```python
from build123d import *

# Parameters (mm, degrees)
PAD011_DEPTH            = 3
FILLET036_R             = 3.35
SKETCH183_R             = 1.15
POCKET052_DEPTH         = 3
POCKET054_DEPTH         = 5
SKETCH187_W             = 31
SKETCH187_H             = 20
POCKET055_DEPTH         = 1.5
BODY023_ROLL_ANGLE      = 180
BODY023_PLACEMENT_ANGLE = -90


with BuildPart() as part:
    # Sketch182 → Pad011 (new body)
    with BuildSketch(Plane(origin=(0, 0, 0), x_dir=(1, 0, 0), z_dir=(0, 0, -1))):
        Polygon((101.467362, -402.500006), (130.400002, -402.500006), (135.400002, -402.500006), (135.400002, -397.500006), (174.999975, -357.90402), (174.999975, -245), (289.999995, -245), (294.999995, -245), (294.999995, -215), (289.999995, -215), (224.999995, -215), (224.999995, -199.999997), (219.999995, -199.999997), (199.999995, -199.999997), (194.999995, -199.999997), (194.999995, -215.000003), (168.459985, -215.000003), (161.999993, -198.359996), (161.999993, -115.000006), (161.999993, -110.000006), (156.999993, -110.000006), (134.576923, -122.534363), (131.999997, -126.895911), (131.999997, -200.027011), (144.989344, -239.967928), (144.989344, -343.839368), (96.467362, -392.500006), (96.467362, -397.500006), (96.467362, -402.500006), align=None)
    extrude(amount=PAD011_DEPTH)

    # Fillet036
    fillet036_edges = [part.edges().sort_by_distance(p)[0] for p in [
        (194.999995, 215.000003, -1.5),
        (168.459985, 215.000003, -1.5),
        (161.999993, 198.359996, -1.5),
        (161.999993, 110.000006, -1.5),
        (156.999993, 110.000006, -1.5),
        (134.576923, 122.534363, -1.5),
        (131.999997, 126.895911, -1.5),
        (131.999997, 200.027011, -1.5),
        (144.989344, 239.967928, -1.5),
        (144.989344, 343.839368, -1.5),
        (96.467362, 392.500006, -1.5),
        (135.400002, 397.500006, -1.5),
        (174.999975, 357.90402, -1.5),
        (174.999975, 245, -1.5),
        (294.999995, 245, -1.5),
        (294.999995, 215, -1.5),
        (224.999995, 215, -1.5),
    ]]
    fillet(fillet036_edges, radius=FILLET036_R)

    # Sketch183 (on Face5 of Fillet036) → Pocket052 (cut)
    with BuildSketch(Plane(origin=(0, 0, -3), x_dir=(1, 0, 0), z_dir=(0, 0, -1))):
        with Locations((105, -389)):
            Circle(SKETCH183_R)
        with Locations((145, -349)):
            Circle(SKETCH183_R)
        with Locations((147.500002, -309.000005)):
            Circle(SKETCH183_R)
        with Locations((147.500002, -259.000004)):
            Circle(SKETCH183_R)
        with Locations((172.500003, -259.000004)):
            Circle(SKETCH183_R)
        with Locations((172.500003, -309.000005)):
            Circle(SKETCH183_R)
        with Locations((172.500003, -349.000005)):
            Circle(SKETCH183_R)
        with Locations((147.665007, -382.765018)):
            Circle(SKETCH183_R)
        with Locations((178.000003, -242.500004)):
            Circle(SKETCH183_R)
        with Locations((218.000003, -242.500004)):
            Circle(SKETCH183_R)
        with Locations((258.000004, -242.500004)):
            Circle(SKETCH183_R)
        with Locations((258.000004, -217.500003)):
            Circle(SKETCH183_R)
        with Locations((292, -242.500004)):
            Circle(SKETCH183_R)
        with Locations((292.000004, -217.500003)):
            Circle(SKETCH183_R)
        with Locations((292.500004, -230.000003)):
            Circle(SKETCH183_R)
        with Locations((223.000003, -217.000003)):
            Circle(SKETCH183_R)
        with Locations((197, -217)):
            Circle(SKETCH183_R)
        with Locations((166.109996, -217.109995)):
            Circle(SKETCH183_R)
        with Locations((147.500002, -239)):
            Circle(SKETCH183_R)
        with Locations((141, -220)):
            Circle(SKETCH183_R)
        with Locations((134.427551, -201)):
            Circle(SKETCH183_R)
        with Locations((160.149996, -200.999996)):
            Circle(SKETCH183_R)
        with Locations((134.427551, -161)):
            Circle(SKETCH183_R)
        with Locations((159.500002, -161.000002)):
            Circle(SKETCH183_R)
        with Locations((137, -124)):
            Circle(SKETCH183_R)
        with Locations((146.849997, -118.149997)):
            Circle(SKETCH183_R)
        with Locations((159, -113)):
            Circle(SKETCH183_R)
    extrude(amount=-POCKET052_DEPTH, mode=Mode.SUBTRACT)

    # Sketch186 (on Face5 of Pocket052) → Pocket054 (cut)
    with BuildSketch(Plane(origin=(0, 0, -3), x_dir=(1, 0, 0), z_dir=(0, 0, -1))):
        Polygon((175, -249), (130, -249), (130, -100), (170, -100), (170, -190), (300, -190), (300, -249), align=None)
    extrude(amount=-POCKET054_DEPTH, mode=Mode.SUBTRACT)

    # Sketch187 (on Face25 of Pocket054) → Pocket055 (cut)
    with BuildSketch(Plane(origin=(0, 0, -3), x_dir=(1, 0, 0), z_dir=(0, 0, -1))):
        with Locations((159.5, -259)):
            Rectangle(SKETCH187_W, SKETCH187_H)
    extrude(amount=-POCKET055_DEPTH, mode=Mode.SUBTRACT)


with BuildPart() as part_1:
    # Body023 roll: moved
    add(part.part.rotate(Axis((0, 0, 0), (1, 0, 0)), BODY023_ROLL_ANGLE))


with BuildPart() as part_2:
    # Body023 placement: moved
    add(part_1.part.moved(Location((0, 0, -5))).rotate(Axis((0, 0, -5), (0, 0, 1)), BODY023_PLACEMENT_ANGLE))


solid = part_2.part
```
Check sheet for the modelled part. Datum: model origin and axes. Units: mm. A direction names the side the tool comes from. Coordinates: 2 decimals unless noted, no trailing zeros. Loops run counter-clockwise (first coordinate to the right, second up) from the corner with the lowest first, then second, coordinate; pieces in that order, holes last. Notation, with made-up numbers: M 80,-16.75 L 87,-16.75 A19 cw 87,20.25 Z; hole C 6,78.5 d1. An arc over 180 degrees is marked long. Answer as a JSON object with one key per item and string values.
1. Sectioned sample at A-A on z = -3. Record the cut outline in (x, y) (3 decimals), and give its area (3 significant figures).
Outcome:
{"outline": "M -402.5,-135.4 L -398.888,-135.4 A3.35 cw -396.519,-136.381 L -358.885,-174.019 A3.35 ccw -356.516,-175 L -269,-175 L -269,-144.989 L -342.455,-144.989 A3.35 cw -344.82,-144.012 L -391.519,-97.445 A3.35 ccw -393.885,-96.467 L -402.5,-96.467 Z; hole C -389,-105 d2.3; hole C -382.765,-147.665 d2.3; hole C -349,-172.5 d2.3; hole C -349,-145 d2.3; hole C -309,-172.5 d2.3; hole C -309,-147.5 d2.3", "area": "4,670 mm²"}
2. Sectioned sample at B-B on y = -160.5. Record the cut outline in (x, z), and give its area (3 significant figures).
Outcome:
{"outline": "M -372.4,-5 L -249,-5 L -249,-3.5 L -269,-3.5 L -269,-2 L -372.4,-2 Z", "area": "340 mm²"}
3. Sectioned sample at C-C on x = -288. Record the cut outline in (y, z), and give its area (3 significant figures).
Outcome:
{"outline": "M -175,-5 L -144.99,-5 L -144.99,-2 L -175,-2 Z", "area": "90.0 mm²"}
4. Depth check by flat-ended pin: P1, Ø1, axis at y = -140, z = -3, coming from the +X side; P2, Ø2, axis at x = -259, y = -147.5, coming from the +Z side; P3, Ø1.5, axis at y = -158, z = -4.5, coming from the -X side; P4, Ø1, axis at y = -150.5, z = -3.5, coming from the -X side. Enter the tip coordinate at first touch or a pass-through.
Outcome:
{"P1": "x = -348.34", "P2": "through", "P3": "x = -375.65", "P4": "x = -382.9"}
5. Sectioned sample at D-D on y = -120. Record the cut outline in (x, z).
Outcome:
{"outline": "M -402.5,-5 L -368.9,-5 L -368.9,-2 L -402.5,-2 Z"}
6. Access from +Z, -Z, +X, -X, +Y, -Y to the whole of each face (thin tool, end or side, straight path). Record for faces 1 (the flat face through (-259, -160, -3.5)), 2 (the flat face through (-401, -135.4, -4)), 3 (the flat face through (-295, -144.989, -4)).
Outcome:
{"face 1": "+Z, +X, +Y, -Y", "face 2": "+Z, -Z, -X, -Y", "face 3": "+Z, -Z, +X, +Y"}
7. Scan lines: L1, parallel to X at y = -147.5, z = -2.45; L2, parallel to Y at x = -349, z = -2.8; L3, parallel to X at y = -172, z = -2.35. Record each from-to range of solid material in increasing order. Write a range as from..to.
Outcome:
{"L1": "-385.4..-383.9, -381.63..-310.15, -307.85..-269", "L2": "-175..-173.65, -171.35..-146.15, -143.85..-139.84", "L3": "-360.9..-350.04, -347.96..-310.04, -307.96..-269"}
